```python
from build123d import *

# Parameters (mm, degrees)
SKETCH_1_W      = 78
SKETCH_1_H      = 40
EXTRUDE_1_DEPTH = 18
SKETCH_2_W      = 4.5
SKETCH_2_H      = 6.35
EXTRUDE_2_DEPTH = 0.2


with BuildPart() as part:
    # 草图1 → 凸台-拉伸1 (new body)
    with BuildSketch(Plane.XY):
        Rectangle(SKETCH_1_W, SKETCH_1_H)
    extrude(amount=EXTRUDE_1_DEPTH)

    # 草图2 → 凸台-拉伸2 (add)
    with BuildSketch(Plane.XY.offset(18)):
        with Locations((-41.25, 9.55)):
            Rectangle(SKETCH_2_W, SKETCH_2_H)
        with Locations((-41.25, -9.55)):
            Rectangle(SKETCH_2_W, SKETCH_2_H)
        with Locations((41.25, 9.55)):
            Rectangle(SKETCH_2_W, SKETCH_2_H)
        with Locations((41.25, -9.55)):
            Rectangle(SKETCH_2_W, SKETCH_2_H)
    extrude(amount=-EXTRUDE_2_DEPTH)


solid = part.part
```
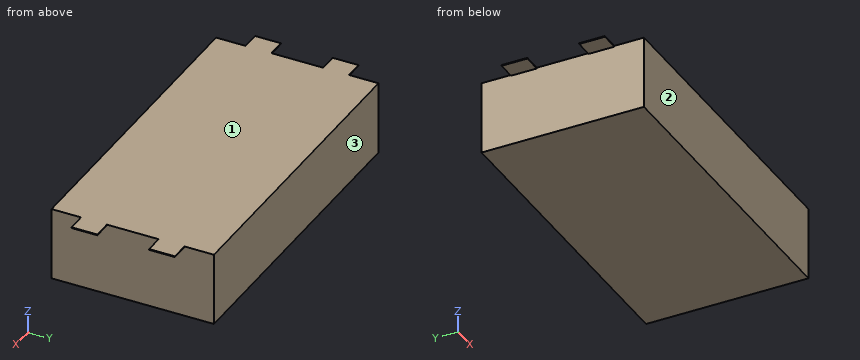
Check sheet for the modelled part. Datum: model origin and axes. Units: mm. Face numbers are marked on the shaded views. Round coordinates to 2 decimals unless told otherwise and drop trailing zeros. Order: outer loops, then holes, each group sorted by start corner. A loop starts at its lowest first (then second) coordinate and runs counter-clockwise, first axis right, second up. Notation, with made-up numbers: (48, 74) -> (96, 74) arc R26 ccw to (96, 113) -> close; hole circle Ø6 at (10.5, 60). An arc over 180 degrees is marked (long way). Use CSV: the item, a comma, the result in double quotes.
(1) Draft check along Y on the marked faces 1, 2 and 3. Enter one of: pulls with the +Y half, pulls with the -Y half, needs draft (parallel to the pull), parting line crosses it, or undercut.
Worked out:
face 1,"needs draft"
face 2,"pulls with the -Y half"
face 3,"pulls with the +Y half"
(2) Cross-section at B-B (z = 1.5). Record the boundary of the cut face in (x, y).
Worked out:
outline,"(-39, -20) -> (39, -20) -> (39, 20) -> (-39, 20) -> close"
(3) Material ranges on line 1 along X through (y, z) = (-16, 8.75), recorded low to high. Write a range as from..to.
Worked out:
line 1,"-39..39"
(4) Depth check by flat-ended pin: pin 1 (2 mm diameter, centred on x = 41.5, y = -10, fed in from -Z); pin 2 (5 mm diameter, centred on y = 13.5, z = 10.5, fed in from -X); pin 3 (3.5 mm diameter, centred on x = -40, y = -10.5, fed in from -Z); pin 4 (5.5 mm diameter, centred on y = 0.5, z = 12.5, fed in from +X). Enter the tip coordinate at first touch or a pass-through.
Worked out:
pin 1,"z = 17.8"
pin 2,"x = -39"
pin 3,"z = 0"
pin 4,"x = 39"
(5) Cross-section at A-A (y = -9). Record the boundary of the cut face in (x, z), and give its area (3 significant figures).
Worked out:
outline,"(-43.5, 17.8) -> (-39, 17.8) -> (-39, 0) -> (39, 0) -> (39, 17.8) -> (43.5, 17.8) -> (43.5, 18) -> (-43.5, 18) -> close"
area,"1,410 mm²"
(6) Cross-section at C-C (y = -2). Record the boundary of the cut face in (x, z).
Worked out:
outline,"(-39, 0) -> (39, 0) -> (39, 18) -> (-39, 18) -> close"
